Geometry check sheet. Reference: drawing and pictorial views, mm from the part's lowest x, y, z. Round coordinates to 2 decimals unless told otherwise and drop trailing zeros. Write each loop counter-clockwise with the first axis right and the second up, starting at its lowest first coordinate (ties: lowest second). Pieces come first, ordered by that corner, then holes. Notation, with made-up numbers: (-22, 44) -> (26, 44) arc R13 cw to (26, 57) -> close; hole circle Ø4 at (41, 32). An arc over 180 degrees is marked (long way). Write item = value, one per line.
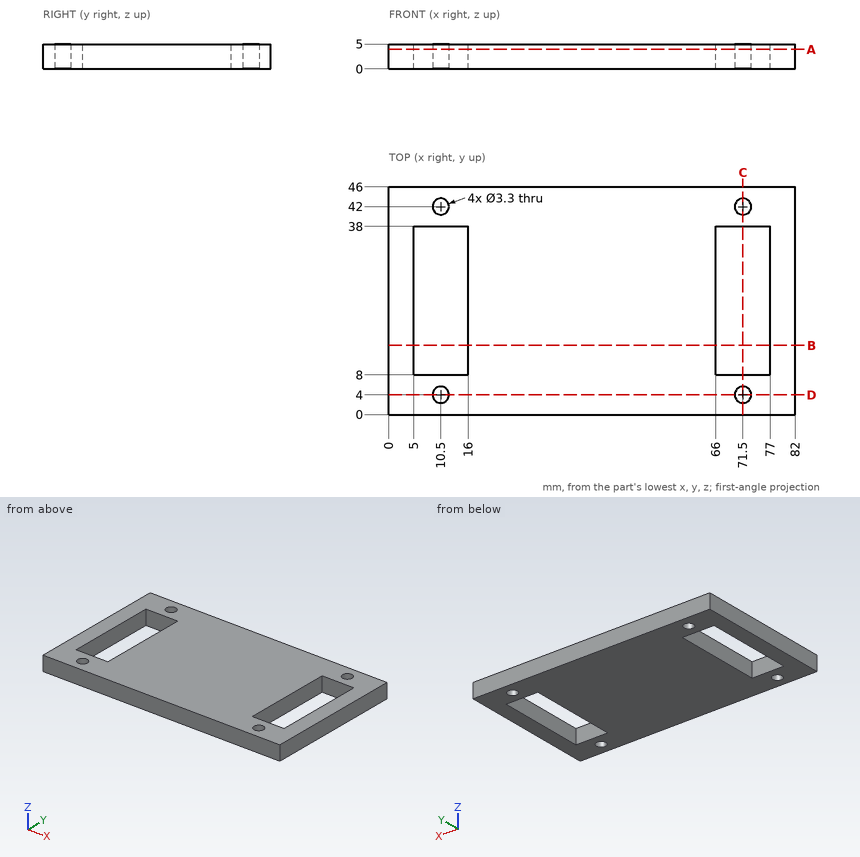
(1) Sectioned sample at D-D on y = 4. Enter the section's corners in (x, z), then the cut area to 3 significant figures.
Worked answers:
outline = (0, 0) -> (8.85, 0) -> (8.85, 5) -> (0, 5) -> close; (12.15, 0) -> (69.85, 0) -> (69.85, 5) -> (12.15, 5) -> close; (73.15, 0) -> (82, 0) -> (82, 5) -> (73.15, 5) -> close
area = 377 mm²
(2) Material ranges on L1, parallel to X at y = 31, z = 0.8; L2, parallel to Y at x = 71.5, z = 1.8; L3, parallel to Y at x = 13, z = 0.35, recorded low to high. Write a range as [from, to].
Worked answers:
L1 = [0, 5], [16, 66], [77, 82]
L2 = [0, 2.35], [5.65, 8], [38, 40.35], [43.65, 46]
L3 = [0, 8], [38, 46]
(3) Sectioned sample at B-B on y = 14. Enter the section's corners in (x, z).
Worked answers:
outline = (0, 0) -> (5, 0) -> (5, 5) -> (0, 5) -> close; (16, 0) -> (66, 0) -> (66, 5) -> (16, 5) -> close; (77, 0) -> (82, 0) -> (82, 5) -> (77, 5) -> close
(4) Sectioned sample at C-C on x = 71.5. Enter the section's corners in (y, z).
Worked answers:
outline = (0, 0) -> (2.35, 0) -> (2.35, 5) -> (0, 5) -> close; (5.65, 0) -> (8, 0) -> (8, 5) -> (5.65, 5) -> close; (38, 0) -> (40.35, 0) -> (40.35, 5) -> (38, 5) -> close; (43.65, 0) -> (46, 0) -> (46, 5) -> (43.65, 5) -> close
(5) Sectioned sample at A-A on z = 3.9. Enter the section's corners in (x, y), then the cut area to 3 significant figures.
Worked answers:
outline = (0, 0) -> (82, 0) -> (82, 46) -> (0, 46) -> close; hole (5, 8) -> (16, 8) -> (16, 38) -> (5, 38) -> close; hole circle Ø3.3 at (10.5, 4); hole circle Ø3.3 at (10.5, 42); hole (66, 8) -> (77, 8) -> (77, 38) -> (66, 38) -> close; hole circle Ø3.3 at (71.5, 4); hole circle Ø3.3 at (71.5, 42)
area = 3,080 mm²
(6) Go/stop test with a flat-tipped pin: P1, Ø3, axis at y = 18, z = 4, coming from the -X side. Record where the tip stops, or that it passes through.
Worked answers:
P1 = 0
